Check sheet for the modelled part. Datum: model origin and axes. Units: mm. A direction names the side the tool comes from. Give positions to 0.01 mm unless a question says otherwise; leave off trailing zeros. Order: outer loops, then holes, each group sorted by start corner. A loop starts at its lowest first (then second) coordinate and runs counter-clockwise, first axis right, second up. Notation, with made-up numbers: (54.25, -29.5) -> (85.25, -29.5) arc R23 ccw to (85.25, -18.5) -> close; hole circle Ø2 at (20.5, -5). An arc over 180 degrees is marked (long way). Answer in a Markdown table with one row per item. Add a question column.
(1) Go/stop test with flat-tipped pins: pin 1 (2.5 mm diameter, centred on y = 132, z = -2.5, fed in from +X); pin 2 (12 mm diameter, centred on x = -17.5, y = -8, fed in from -Z); pin 3 (6 mm diameter, centred on x = 34, z = -3.5, fed in from +Y). Record where each tip stops, or that it passes through.
(2) Cross-section at B-B (x = 10.5). Record the cut outline in (y, z).
(3) Thickness scan on L1, parallel to X at y = -12, z = -7.75; L2, parallel to Z at x = 28.5, y = 13; L3, parallel to Y at x = 22.5, z = -3. Record the ranges inside material, lowest first. Write a range as [from, to].
(4) Release check for a two-part mould opening along Z. For faces 6 (the face through (-36.49, 78.57, -9.79)), 7 (the face through (36, 37, -15.875)), 8 (the face through (21.17, -43.378, -1.655)) record: released by +Z, released by -Z, zero draft, split by the parting line, or undercut.
(5) Set-up check for faces 1 (the face through (35, 124.121, -3)), 2 (the face through (36.45, -43.16, -9.98)), 3 (the face through (34.836, 40, -10)), 4 (the face through (-35, 124.121, -3)), 5 (the face through (0, -47.329, -2)): record each of +Z, -Z, +X, -X, +Y, -Y from which the full face is reachable in a straight line by a thin tool's end or side.
(6) Cross-section at A-A (y = 20.5). Record the cut outline in (x, z) (3 decimals), then the cut area to 3 significant figures.
```python
from build123d import *
from OCP.BRepFilletAPI import BRepFilletAPI_MakeChamfer

# Parameters (mm, degrees)
SKETCH1_W                      = 76.2
SKETCH1_H                      = 171.45
BASE_FLANGE1_DEPTH             = 3.2639
EDGE_FLANGE1_STRIP_W           = 15.5956
EDGE_FLANGE1_STRIP_H           = 3.2639
EDGE_FLANGE1_STRIP_CUT_DEPTH   = 171.45
EDGE_FLANGE1_STRIP_2_W         = 15.5956
EDGE_FLANGE1_STRIP_2_H         = 3.2639
EDGE_FLANGE1_STRIP_CUT_2_DEPTH = 171.45
EDGE_FLANGE1_DEPTH             = 171.45
EDGE_FLANGE1_BEND_DEPTH        = 171.45
F_10_0_1935_DIAMETER_HOLE1_D   = 4.9149
SKETCH33_W                     = 54.4322
SKETCH33_H                     = 15.875
BOSS_EXTRUDE1_DEPTH            = 3.2639
CHAMFER1_SIZE                  = 7.9375
CHAMFER1_SIZE2                 = 6.427660763
F_10_0_1935_DIAMETER_HOLE2_D   = 4.9149
FILLET1_R                      = 3.175


# Sheet-metal steps are written as plain solids
with BuildPart() as part:
    # Sketch1 → Base-Flange1 (new body)
    with BuildSketch(Plane.XY):
        with Locations((0, 38.396418)):
            Rectangle(SKETCH1_W, SKETCH1_H)
    extrude(amount=-BASE_FLANGE1_DEPTH)

    # Edge-Flange1 strip (across the edge) → Edge-Flange1 strip cut (cut)
    with BuildSketch(Plane(origin=(38.1, 124.121418, -3.2639), x_dir=(-1, 0, 0), z_dir=(0, -1, 0))):
        with Locations((-3.2639, -1.63195)):
            Rectangle(EDGE_FLANGE1_STRIP_W, EDGE_FLANGE1_STRIP_H)
    extrude(amount=EDGE_FLANGE1_STRIP_CUT_DEPTH, mode=Mode.SUBTRACT)

    # Edge-Flange1 strip 2 (across the edge) → Edge-Flange1 strip cut 2 (cut)
    with BuildSketch(Plane(origin=(-38.1, -47.328582, -3.2639), x_dir=(1, 0, 0), z_dir=(0, 1, 0))):
        with Locations((-3.2639, -1.63195)):
            Rectangle(EDGE_FLANGE1_STRIP_2_W, EDGE_FLANGE1_STRIP_2_H)
    extrude(amount=EDGE_FLANGE1_STRIP_CUT_2_DEPTH, mode=Mode.SUBTRACT)

    # Edge-Flange1 section (across the edge) → Edge-Flange1 (add)
    with BuildSketch(Plane(origin=(38.1, 124.121418, -3.2639), x_dir=(-1, 0, 0), z_dir=(0, -1, 0))):
        with BuildLine():
            Line((0, 1.27), (0, 12.6111))
            Line((0, 12.6111), (3.2639, 12.6111))
            Line((3.2639, 12.6111), (3.2639, 1.27))
            ThreePointArc((3.2639, 1.27), (3.635874388, 0.371974388), (4.5339, 0))
            Line((4.5339, 0), (4.5339, -3.2639))
            ThreePointArc((4.5339, -3.2639), (1.327948565, -1.935951435), (0, 1.27))
        make_face()
    extrude(amount=EDGE_FLANGE1_DEPTH)

    # Edge-Flange1 section 2 (across the edge) → Edge-Flange1 bend (add)
    with BuildSketch(Plane(origin=(-38.1, -47.328582, -3.2639), x_dir=(1, 0, 0), z_dir=(0, 1, 0))):
        with BuildLine():
            Line((0, 1.27), (0, 12.6111))
            Line((0, 12.6111), (3.2639, 12.6111))
            Line((3.2639, 12.6111), (3.2639, 1.27))
            ThreePointArc((3.2639, 1.27), (3.635874388, 0.371974388), (4.5339, 0))
            Line((4.5339, 0), (4.5339, -3.2639))
            ThreePointArc((4.5339, -3.2639), (1.327948565, -1.935951435), (0, 1.27))
        make_face()
    extrude(amount=EDGE_FLANGE1_BEND_DEPTH)

    # #10 (0.1935) Diameter Hole1 (through all)
    with Locations(Plane(origin=(38.1, 0, 0), x_dir=(0, 0, -1), z_dir=(1, 0, 0))):
        with Locations((11.1125, 76.496418), (11.1125, -40.978582), (11.1125, 111.421418)):
            Hole(F_10_0_1935_DIAMETER_HOLE1_D / 2)

    # Sketch33 → Boss-Extrude1 (add)
    with BuildSketch(Plane.XY):
        with Locations((0, 132.058918)):
            Rectangle(SKETCH33_W, SKETCH33_H)
    extrude(amount=-BOSS_EXTRUDE1_DEPTH)

    # Chamfer1: one chamfer whose edges measure the first distance from different faces: ONE call of the kernel's chamfer builder (chamfer() names one face for all edges)
    chamfer1_edges_1 = [part.edges().sort_by_distance(p)[0] for p in [
        (36.46805, 124.121418, -15.875),
    ]]
    chamfer1_side_1 = [part.faces().sort_by_distance(p)[0] for p in [
        (36.46805, 38.396418, -15.875),
    ]]
    chamfer1_edges_2 = [part.edges().sort_by_distance(p)[0] for p in [
        (-36.46805, 124.121418, -15.875),
    ]]
    chamfer1_side_2 = [part.faces().sort_by_distance(p)[0] for p in [
        (-36.46805, 38.396418, -15.875),
    ]]
    chamfer1 = BRepFilletAPI_MakeChamfer(part.part.solid().wrapped)
    for e in chamfer1_edges_1:
        chamfer1.Add(CHAMFER1_SIZE, CHAMFER1_SIZE2, e.wrapped, chamfer1_side_1[0].wrapped)  # the first distance lies on this face
    for e in chamfer1_edges_2:
        chamfer1.Add(CHAMFER1_SIZE, CHAMFER1_SIZE2, e.wrapped, chamfer1_side_2[0].wrapped)  # the first distance lies on this face
    add(Compound.cast(chamfer1.Shape()), mode=Mode.REPLACE)

    # #10 (0.1935) Diameter Hole2 (through all)
    with Locations(Plane.XY):
        with Locations((-20.6375, -40.978582), (20.6375, -40.978582)):
            Hole(F_10_0_1935_DIAMETER_HOLE2_D / 2)

    # Fillet1
    fillet1_edges = [part.edges().sort_by_distance(p)[0] for p in [
        (-27.2161, 124.121418, -1.63195),
        (-27.2161, 139.996418, -1.63195),
        (27.2161, 139.996418, -1.63195),
        (27.2161, 124.121418, -1.63195),
        (-36.46805, 116.183918, -15.875),
        (-36.46805, 124.121418, -9.447339237),
        (36.46805, 124.121418, -9.447339237),
        (36.46805, 116.183918, -15.875),
        (36.46805, -47.328582, -15.875),
        (-36.46805, -47.328582, -15.875),
    ]]
    fillet(fillet1_edges, radius=FILLET1_R)


solid = part.part
```
Answer below:
| question | item | result |
|---|---|---|
| 1 | pin 1 | stops at x = 27.22 |
| 1 | pin 2 | stops at z = -3.26 |
| 1 | pin 3 | stops at y = 124.12 |
| 2 | outline | (-47.33, -3.26) -> (140, -3.26) -> (140, 0) -> (-47.33, 0) -> close |
| 3 | L1 | x = [-38.1, -34.84], [34.84, 38.1] |
| 3 | L2 | z = [-3.26, 0] |
| 3 | L3 | y = [-47.33, -42.58], [-39.38, 140] |
| 4 | face 6 | undercut |
| 4 | face 7 | released by -Z |
| 4 | face 8 | zero draft |
| 5 | face 1 | +Z, -Z, +X, +Y |
| 5 | face 2 | +X, -X |
| 5 | face 3 | -Z, +Y, -Y |
| 5 | face 4 | +Z, -Z, -X, +Y |
| 5 | face 5 | +Z, -Z, +X, -X, -Y |
| 6 | outline | (-38.1, -15.875) -> (-34.836, -15.875) -> (-34.836, -4.534) arc R1.27 cw to (-33.566, -3.264) -> (33.566, -3.264) arc R1.27 cw to (34.836, -4.534) -> (34.836, -15.875) -> (38.1, -15.875) -> (38.1, -4.534) arc R4.534 ccw to (33.566, 0) -> (-33.566, 0) arc R4.534 ccw to (-38.1, -4.534) -> close |
| 6 | area | 323 mm² |
